The drawing under review shows one solid part. Ordinate dimensions are in mm from its lowest x, y, z. A direction names the side the tool comes from. Give positions to 0.01 mm unless a question says otherwise; leave off trailing zeros. Order: outer loops, then holes, each group sorted by start corner. A loop starts at its lowest first (then second) coordinate and runs counter-clockwise, first axis right, second up. Notation, with made-up numbers: (-26, 69) -> (3, 69) arc R23 ccw to (3, 103) -> close; hole circle Ø9 at (1.25, 59.25). An arc over 180 degrees is marked (long way). Return JSON: item names as keys, results as strings. Group by question number.
1) Insertion check: P1, Ø8, axis at y = 10, z = 22.5, coming from the -X side; P2, Ø3, axis at x = 26, y = 10, coming from the +Z side; P3, Ø10, axis at y = 21.5, z = 8, coming from the +X side; P4, Ø1.3, axis at y = 11, z = 14, coming from the -X side. Each pin has a flat end and moves straight along its axis. Give the tip position at first contact, or say it passes through.
2) Add section C-C (y = 14). Give the boundary of the cut face in (x, z).
3) The part is to be moulded in two halves that separate along Y. For the marked faces 1, 2, 3 and 4, say which applies: released by +Y, released by -Y, zero draft, split by the parting line, or undercut.
4) To check wall thickness, follow line 1 along Y through (x, z) = (10, 21.75); line 2 along Z through (x, y) = (3.5, 15); line 3 along Z through (x, y) = (35, 3.5) (1 decimal). State the ranges of each line that lie inside material, in increasing order.
5) Add section A-A (z = 21). Give the boundary of the cut face in (x, y).
6) Add section B-B (x = 13). Give the boundary of the cut face in (y, z), then the cut area to 3 significant figures.
7) For the marked faces 5 and 6, list the 3-axis set-ups (+Z, -Z, +X, -X, +Y, -Y) from which the entire face can be reached by the end or side of a thin tool; tool diameter is ignored.
8) Add section D-D (z = 13.25). Give the boundary of the cut face in (x, y).
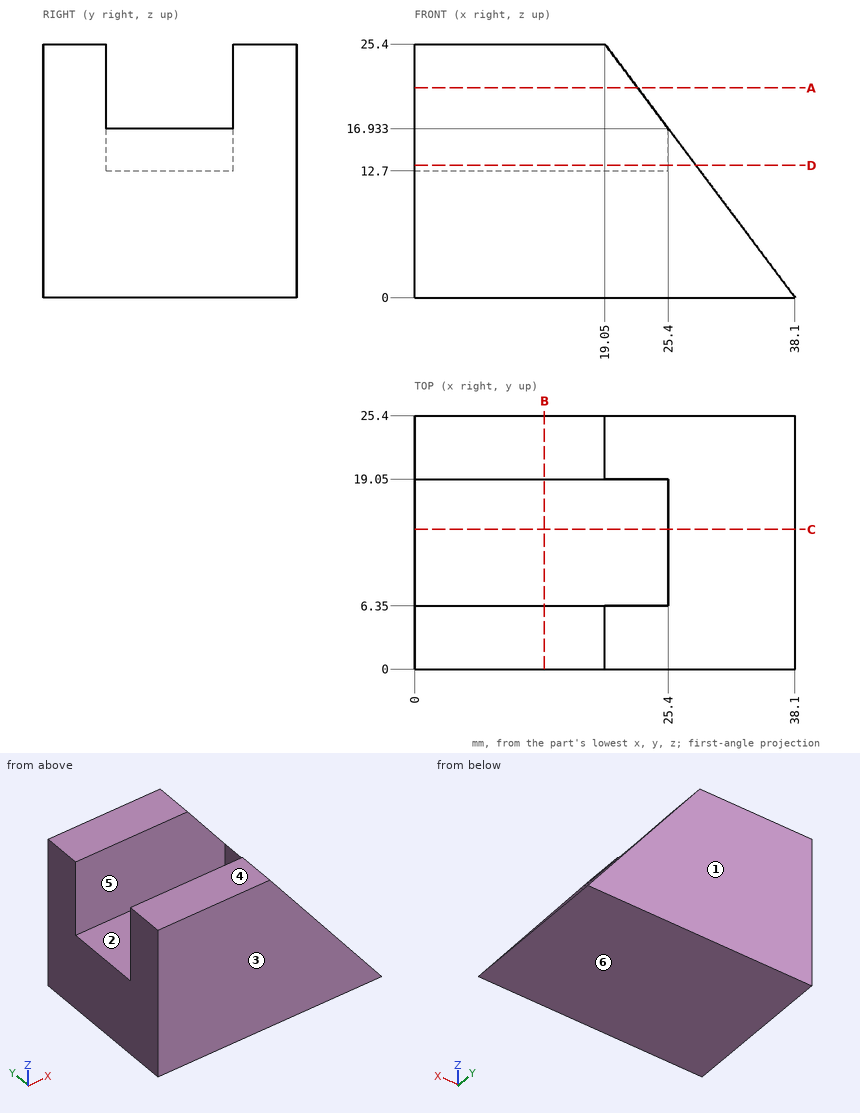
Evaluation:
{
 "1": {"P1": "x = 0", "P2": "z = 16.93", "P3": "x = 35.85", "P4": "x = 25.4"},
 "2": {"outline": "(0, 0) -> (38.1, 0) -> (25.4, 16.93) -> (25.4, 12.7) -> (0, 12.7) -> close"},
 "3": {"face 1": "released by +Y", "face 2": "undercut", "face 3": "released by -Y", "face 4": "zero draft"},
 "4": {"line 1": "0 to 6.35, 19.05 to 25.4", "line 2": "0 to 12.7", "line 3": "0 to 4.1"},
 "5": {"outline": "(0, 0) -> (22.35, 0) -> (22.35, 6.35) -> (0, 6.35) -> close; (0, 19.05) -> (22.35, 19.05) -> (22.35, 25.4) -> (0, 25.4) -> close"},
 "6": {"outline": "(0, 0) -> (25.4, 0) -> (25.4, 25.4) -> (19.05, 25.4) -> (19.05, 12.7) -> (6.35, 12.7) -> (6.35, 25.4) -> (0, 25.4) -> close", "area": "484 mm^2"},
 "7": {"face 5": "+Z, -X", "face 6": "-Z, +X, -X, +Y, -Y"},
 "8": {"outline": "(0, 0) -> (28.16, 0) -> (28.16, 25.4) -> (0, 25.4) -> (0, 19.05) -> (25.4, 19.05) -> (25.4, 6.35) -> (0, 6.35) -> close"}
}
